Geometry: final body of the model. Coordinates: model frame, mm. A direction names the side the tool comes from. Give positions to 0.01 mm unless a question says otherwise; leave off trailing zeros. Write each loop counter-clockwise with the first axis right and the second up, starting at its lowest first coordinate (ties: lowest second). Pieces come first, ordered by that corner, then holes.
Q1. Reachability of faces 5 (the face through (-12.894, -149.265, 3.944)), 6 (the face through (-113.6, -17.8, 5.7)) from +Z, -Z, +X, -X, +Y, -Y: full face, straight path, thin tool, end or side. Return the list, or none.
Q2. Cut plane A-A on x = -139.75. Return the cut outline in (y, z), plus the area to 3 significant figures.
Q3. Draft query along X for faces 1 (the face through (12.72, -148.95, 3.94)), 2 (the face through (-230.87, 202.38, 4.06)), 3 (the face through (-169.77, -10.2, 6.99)), 4 (the face through (231.13, 202.12, 4.06)). Return one class per face: pulls with the +X half, pulls with the -X half, needs draft (parallel to the pull), parting line crosses it, or undercut.
Q4. Line query: L1, parallel to Y at x = 0, z = 4.75; L2, parallel to Y at x = 183.25, z = 2.25; L3, parallel to X at y = 137.5, z = 3.75. Output: solid intervals per line, ascending.
Q5. Pin query (flat end, axial travel): pin 1 (4 mm diameter, centred on x = 147.5, z = 5, fed in from +Y); pin 2 (2.5 mm diameter, centred on y = 43, z = 3.5, fed in from +X); pin 3 (2 mm diameter, centred on x = 109.75, y = 59.25, fed in from +Z); pin 4 (4 mm diameter, centred on x = 223, z = 3.5, fed in from -Y). Return the tip coordinate at first contact, or that it passes through.
Q6. Cut plane B-B on y = -5. Count the separate pieces of the cut face and the enclosed holes in it, plus the area to 3 significant figures.
```python
from build123d import *

# Parameters (mm, degrees)
BOSS_EXTRUDE1_DEPTH        = 8
F_6_5_6_5_DIAMETER_HOLE1_D = 6.5
CUT_EXTRUDE1_DEPTH         = 325.495088493
CUT_EXTRUDE6_REACH         = 326.495
CUT_EXTRUDE7_REACH         = 326.495
CUT_EXTRUDE5_REACH         = 326.495
SKETCH9_R                  = 32.5
CHAMFER1_SIZE              = 9
CHAMFER1_SIZE2             = 6
CUT_EXTRUDE8_REACH         = 326.495
SKETCH13_R                 = 1.6
CUT_EXTRUDE9_REACH         = 326.495
CUT_EXTRUDE10_DEPTH        = 325.495088493
CUT_EXTRUDE11_REACH        = 326.495
SKETCH16_R                 = 1.25


with BuildPart() as part:
    # Sketch1 → Boss-Extrude1 (new body)
    with BuildSketch(Plane.XY.offset(8)):
        with BuildLine():
            Line((152.5, 201.25), (137.5, 201.25))
            ThreePointArc((137.5, 201.25), (135.586582838, 201.630602337), (133.964466094, 202.714466094))
            Line((133.964466094, 202.714466094), (125.428932188, 211.25))
            Line((125.428932188, 211.25), (-222, 211.25))
            Line((-222, 211.25), (-240, 193.25))
            Line((-240, 193.25), (-240, -193.249999907))
            Line((-240, -193.249999907), (-215.000000007, -218.249999899))
            Line((-215.000000007, -218.249999899), (203.5, -218.249999899))
            Line((203.5, -218.249999899), (208.5, -213.249999899))
            Line((208.5, -213.249999899), (208.5, -157.249999899))
            ThreePointArc((208.5, -157.249999899), (209.085786438, -155.835786337), (210.5, -155.249999899))
            Line((210.5, -155.249999899), (235, -155.249999899))
            Line((235, -155.249999899), (240, -150.249999899))
            Line((240, -150.249999899), (240, 8.5))
            ThreePointArc((240, 8.5), (238.828427125, 11.328427125), (236, 12.5))
            Line((236, 12.5), (226, 12.5))
            ThreePointArc((226, 12.5), (223.171572875, 13.671572875), (222, 16.5))
            Line((222, 16.5), (222, 53.5))
            ThreePointArc((222, 53.5), (223.171572875, 56.328427125), (226, 57.5))
            Line((226, 57.5), (236, 57.5))
            ThreePointArc((236, 57.5), (238.828427125, 58.671572875), (240, 61.5))
            Line((240, 61.5), (240, 193.25))
            Line((240, 193.25), (222, 211.25))
            Line((222, 211.25), (164.571067812, 211.25))
            Line((164.571067812, 211.25), (156.035533906, 202.714466094))
            ThreePointArc((156.035533906, 202.714466094), (154.413417162, 201.630602337), (152.5, 201.25))
        make_face()
    extrude(amount=-BOSS_EXTRUDE1_DEPTH)

    # Ø6.5 (6.5) Diameter Hole1 (through all)
    with Locations(Plane.XY.offset(8)):
        with Locations((198.5, -182.25), (0, 182.25), (-198.5, -182.25), (198.5, 182.25), (-198.5, 182.25)):
            Hole(F_6_5_6_5_DIAMETER_HOLE1_D / 2)

    # Sketch4 → Cut-Extrude1 (cut, through all)
    with BuildSketch(Plane(origin=(0, 0, 0), x_dir=(-1, 0, 0), z_dir=(0, 0, -1))):
        with BuildLine():
            Line((-6.556179571, -137.857678016), (-19.056179571, -160.357678016))
            ThreePointArc((-19.056179571, -160.357678016), (-18.964031825, -167.803457974), (-12.5, -171.5))
            Line((-12.5, -171.5), (12.5, -171.5))
            ThreePointArc((12.5, -171.5), (18.964031825, -167.803457974), (19.056179571, -160.357678016))
            Line((19.056179571, -160.357678016), (6.556179571, -137.857678016))
            ThreePointArc((6.556179571, -137.857678016), (0, -134), (-6.556179571, -137.857678016))
        make_face()
    extrude(amount=-CUT_EXTRUDE1_DEPTH, mode=Mode.SUBTRACT)

    # Sketch12 → Cut-Extrude6 (cut, up to next)
    with BuildSketch(Plane(origin=(0, 0, 0), x_dir=(-1, 0, 0), z_dir=(0, 0, -1)), mode=Mode.PRIVATE) as cut_extrude6_sk1:
        with BuildLine():
            Line((103.75, 153.25), (175.75, 153.25))
            ThreePointArc((175.75, 153.25), (179.992640687, 151.492640687), (181.75, 147.25))
            Line((181.75, 147.25), (181.75, 75.25))
            ThreePointArc((181.75, 75.25), (179.992640687, 71.007359313), (175.75, 69.25))
            Line((175.75, 69.25), (103.75, 69.25))
            ThreePointArc((103.75, 69.25), (99.507359313, 71.007359313), (97.75, 75.25))
            Line((97.75, 75.25), (97.75, 147.25))
            ThreePointArc((97.75, 147.25), (99.507359313, 151.492640687), (103.75, 153.25))
        make_face()
    cut_extrude6_tool1 = extrude(cut_extrude6_sk1.sketch, amount=-CUT_EXTRUDE6_REACH, mode=Mode.PRIVATE) & part.part
    # Sketch12 → Cut-Extrude6 (cut, up to next)
    with BuildSketch(Plane(origin=(0, 0, 0), x_dir=(-1, 0, 0), z_dir=(0, 0, -1)), mode=Mode.PRIVATE) as cut_extrude6_sk2:
        with BuildLine():
            Line((123, 12.75), (157.5, 12.75))
            ThreePointArc((157.5, 12.75), (159.621320344, 11.871320344), (160.5, 9.75))
            Line((160.5, 9.75), (160.5, -15))
            ThreePointArc((160.5, -15), (159.621320344, -17.121320344), (157.5, -18))
            Line((157.5, -18), (123, -18))
            ThreePointArc((123, -18), (120.878679656, -17.121320344), (120, -15))
            Line((120, -15), (120, 9.75))
            ThreePointArc((120, 9.75), (120.878679656, 11.871320344), (123, 12.75))
        make_face()
    cut_extrude6_tool2 = extrude(cut_extrude6_sk2.sketch, amount=-CUT_EXTRUDE6_REACH, mode=Mode.PRIVATE) & part.part
    cut_extrude6_1 = cut_extrude6_tool1.solids().sort_by_distance((-139.75, 111.25, 0))[0]
    add(cut_extrude6_1, mode=Mode.SUBTRACT)
    cut_extrude6_2 = cut_extrude6_tool2.solids().sort_by_distance((-140.25, -2.625, 0))[0]
    add(cut_extrude6_2, mode=Mode.SUBTRACT)
    cut_extrude6 = cut_extrude6_1 + cut_extrude6_2  # Cut-Extrude6 as one shape, for the pattern or mirror that repeats it

    # Mirror1: Cut-Extrude6 across plane
    add(cut_extrude6.mirror(Plane(origin=(0, 0, 0), x_dir=(0, 0, 1), z_dir=(1, 0, 0))), mode=Mode.SUBTRACT)

    # Sketch11 → Cut-Extrude7 (cut, up to next)
    with BuildSketch(Plane(origin=(0, 0, 0), x_dir=(-1, 0, 0), z_dir=(0, 0, -1)), mode=Mode.PRIVATE) as cut_extrude7_sk1:
        with BuildLine():
            Line((-2.75, 133.25), (2.75, 133.25))
            ThreePointArc((2.75, 133.25), (6.285533906, 131.785533906), (7.75, 128.25))
            Line((7.75, 128.25), (7.75, 104.25))
            ThreePointArc((7.75, 104.25), (6.285533906, 100.714466094), (2.75, 99.25))
            Line((2.75, 99.25), (-2.75, 99.25))
            ThreePointArc((-2.75, 99.25), (-6.285533906, 100.714466094), (-7.75, 104.25))
            Line((-7.75, 104.25), (-7.75, 128.25))
            ThreePointArc((-7.75, 128.25), (-6.285533906, 131.785533906), (-2.75, 133.25))
        make_face()
    cut_extrude7_tool1 = extrude(cut_extrude7_sk1.sketch, amount=-CUT_EXTRUDE7_REACH, mode=Mode.PRIVATE) & part.part
    # Sketch11 → Cut-Extrude7 (cut, up to next)
    with BuildSketch(Plane(origin=(0, 0, 0), x_dir=(-1, 0, 0), z_dir=(0, 0, -1)), mode=Mode.PRIVATE) as cut_extrude7_sk2:
        with BuildLine():
            Line((-201.75, 116.75), (-194.25, 116.75))
            ThreePointArc((-194.25, 116.75), (-191.421572875, 115.578427125), (-190.25, 112.75))
            Line((-190.25, 112.75), (-190.25, 75.25))
            ThreePointArc((-190.25, 75.25), (-191.421572875, 72.421572875), (-194.25, 71.25))
            Line((-194.25, 71.25), (-201.75, 71.25))
            ThreePointArc((-201.75, 71.25), (-204.578427125, 72.421572875), (-205.75, 75.25))
            Line((-205.75, 75.25), (-205.75, 112.75))
            ThreePointArc((-205.75, 112.75), (-204.578427125, 115.578427125), (-201.75, 116.75))
        make_face()
    cut_extrude7_tool2 = extrude(cut_extrude7_sk2.sketch, amount=-CUT_EXTRUDE7_REACH, mode=Mode.PRIVATE) & part.part
    add(cut_extrude7_tool1.solids().sort_by_distance((0, 116.25, 0))[0], mode=Mode.SUBTRACT)
    add(cut_extrude7_tool2.solids().sort_by_distance((198, 94, 0))[0], mode=Mode.SUBTRACT)

    # Sketch9 → Cut-Extrude5 (cut, up to next)
    with BuildSketch(Plane(origin=(0, 0, 0), x_dir=(-1, 0, 0), z_dir=(0, 0, -1)), mode=Mode.PRIVATE) as cut_extrude5_sk1:
        with Locations((139.75, 2.25)):
            Circle(SKETCH9_R)
    cut_extrude5_tool1 = extrude(cut_extrude5_sk1.sketch, amount=-CUT_EXTRUDE5_REACH, mode=Mode.PRIVATE) & part.part
    add(cut_extrude5_tool1.solids().sort_by_distance((-139.75, 2.25, 0))[0], mode=Mode.SUBTRACT)

    # Chamfer1
    chamfer1_edges = [part.edges().sort_by_distance(p)[0] for p in [
        (-107.25, 2.25, 0),
    ]]
    chamfer1_side = [part.faces().sort_by_distance(p)[0] for p in [
        (-2.503127198, -10.867495519, 0),
    ]]
    chamfer(chamfer1_edges, length=CHAMFER1_SIZE, length2=CHAMFER1_SIZE2, reference=chamfer1_side[0])

    # Sketch13 → Cut-Extrude8 (cut, up to next)
    with BuildSketch(Plane.XY.offset(8), mode=Mode.PRIVATE) as cut_extrude8_sk1:
        with Locations((171, -129)):
            Circle(SKETCH13_R)
    cut_extrude8_tool1 = extrude(cut_extrude8_sk1.sketch, amount=-CUT_EXTRUDE8_REACH, mode=Mode.PRIVATE) & part.part
    # Sketch13 → Cut-Extrude8 (cut, up to next)
    with BuildSketch(Plane.XY.offset(8), mode=Mode.PRIVATE) as cut_extrude8_sk2:
        with Locations((183.25, -186.6)):
            Circle(SKETCH13_R)
    cut_extrude8_tool2 = extrude(cut_extrude8_sk2.sketch, amount=-CUT_EXTRUDE8_REACH, mode=Mode.PRIVATE) & part.part
    add(cut_extrude8_tool1.solids().sort_by_distance((171, -129, 8))[0], mode=Mode.SUBTRACT)
    add(cut_extrude8_tool2.solids().sort_by_distance((183.25, -186.6, 8))[0], mode=Mode.SUBTRACT)

    # Sketch14 → Cut-Extrude9 (cut, up to next)
    with BuildSketch(Plane.XY.offset(8), mode=Mode.PRIVATE) as cut_extrude9_sk1:
        with BuildLine():
            Line((8, 245.685058497), (8, 196.25))
            ThreePointArc((8, 196.25), (0, 188.25), (-8, 196.25))
            Line((-8, 196.25), (-8, 245.685058497))
            ThreePointArc((-8, 245.685058497), (0, 253.685058497), (8, 245.685058497))
        make_face()
    cut_extrude9_tool1 = extrude(cut_extrude9_sk1.sketch, amount=-CUT_EXTRUDE9_REACH, mode=Mode.PRIVATE) & part.part
    add(cut_extrude9_tool1.solids().sort_by_distance((0, 220.967529, 8))[0], mode=Mode.SUBTRACT)

    # Sketch15 → Cut-Extrude10 (cut, through all)
    with BuildSketch(Plane(origin=(0, 0, 0), x_dir=(-1, 0, 0), z_dir=(0, 0, -1))):
        with BuildLine():
            Line((-240, -153.249999899), (-240, -218.249999899))
            Line((-240, -218.249999899), (-207, -218.249999899))
            Line((-207, -218.249999899), (-207, -156.749999899))
            ThreePointArc((-207, -156.749999899), (-208.025126266, -154.275126165), (-210.5, -153.249999899))
            Line((-210.5, -153.249999899), (-240, -153.249999899))
        make_face()
    extrude(amount=-CUT_EXTRUDE10_DEPTH, mode=Mode.SUBTRACT)

    # Sketch16 → Cut-Extrude11 (cut, up to next)
    with BuildSketch(Plane(origin=(0, 0, 0), x_dir=(-1, 0, 0), z_dir=(0, 0, -1)), mode=Mode.PRIVATE) as cut_extrude11_sk1:
        with Locations((-169.75, 59.25)):
            Circle(SKETCH16_R)
    cut_extrude11_tool1 = extrude(cut_extrude11_sk1.sketch, amount=-CUT_EXTRUDE11_REACH, mode=Mode.PRIVATE) & part.part
    # Sketch16 → Cut-Extrude11 (cut, up to next)
    with BuildSketch(Plane(origin=(0, 0, 0), x_dir=(-1, 0, 0), z_dir=(0, 0, -1)), mode=Mode.PRIVATE) as cut_extrude11_sk2:
        with Locations((-109.75, 59.25)):
            Circle(SKETCH16_R)
    cut_extrude11_tool2 = extrude(cut_extrude11_sk2.sketch, amount=-CUT_EXTRUDE11_REACH, mode=Mode.PRIVATE) & part.part
    # Sketch16 → Cut-Extrude11 (cut, up to next)
    with BuildSketch(Plane(origin=(0, 0, 0), x_dir=(-1, 0, 0), z_dir=(0, 0, -1)), mode=Mode.PRIVATE) as cut_extrude11_sk3:
        with BuildLine():
            Line((-182.75, -32.25), (-96.75, -32.25))
            ThreePointArc((-96.75, -32.25), (-95.335786438, -32.835786438), (-94.75, -34.25))
            Line((-94.75, -34.25), (-94.75, -55.25))
            ThreePointArc((-94.75, -55.25), (-95.335786438, -56.664213562), (-96.75, -57.25))
            Line((-96.75, -57.25), (-182.75, -57.25))
            ThreePointArc((-182.75, -57.25), (-184.164213562, -56.664213562), (-184.75, -55.25))
            Line((-184.75, -55.25), (-184.75, -34.25))
            ThreePointArc((-184.75, -34.25), (-184.164213562, -32.835786438), (-182.75, -32.25))
        make_face()
    cut_extrude11_tool3 = extrude(cut_extrude11_sk3.sketch, amount=-CUT_EXTRUDE11_REACH, mode=Mode.PRIVATE) & part.part
    add(cut_extrude11_tool1.solids().sort_by_distance((169.75, 59.25, 0))[0], mode=Mode.SUBTRACT)
    add(cut_extrude11_tool2.solids().sort_by_distance((109.75, 59.25, 0))[0], mode=Mode.SUBTRACT)
    add(cut_extrude11_tool3.solids().sort_by_distance((139.75, -44.75, 0))[0], mode=Mode.SUBTRACT)


solid = part.part
```
Data:
1. face 5: +Z, -Z
1. face 6: -Z
2. outline: (-218.25, 0) - (-39.25, 0) - (-30.25, 6) - (-30.25, 8) - (-218.25, 8) - close; (34.75, 6) - (43.75, 0) - (69.25, 0) - (69.25, 8) - (34.75, 8) - close; (153.25, 0) - (211.25, 0) - (211.25, 8) - (153.25, 8) - close
2. area: 2,190 mm2
3. face 1: undercut
3. face 2: pulls with the -X half
3. face 3: undercut
3. face 4: pulls with the +X half
4. L1: y = -218.25 to -171.5, -134 to 99.25, 133.25 to 179, 185.5 to 188.25
4. L2: y = -218.25 to -188.2, -185 to -57.19, -32.31 to 211.25
4. L3: x = -240 to -181.75, -97.75 to 97.75, 181.75 to 240
5. pin 1: stops at y = 201.25
5. pin 2: stops at x = 222
5. pin 3: passes through
5. pin 4: stops at y = -153.25
6. separate pieces: 3
6. enclosed holes: 0
6. area: 2,950 mm2
